Work out the finished part from the listing and answer in its coordinate system (mm). Round coordinates to 2 decimals unless told otherwise and drop trailing zeros. Write each loop counter-clockwise with the first axis right and the second up, starting at its lowest first coordinate (ties: lowest second). Pieces come first, ordered by that corner, then holes. Notation, with made-up numbers: (36.25, -20) - (40.25, -20) arc R33 cw to (40.25, 8) - close; hole circle Ø10 at (44.5, 49). An arc over 180 degrees is marked (long way). Write item = value, one per line. Start each with the question number.
from build123d import *

# Parameters (mm, degrees)
SKETCH1_W           = 51
SKETCH1_H           = 46
BOSS_EXTRUDE1_DEPTH = 11
FILLET2_R           = 5.5
FILLET3_R           = 5.5


with BuildPart() as part:
    # Sketch1 → Boss-Extrude1 (new body)
    with BuildSketch(Plane.XY):
        Rectangle(SKETCH1_W, SKETCH1_H)
    extrude(amount=BOSS_EXTRUDE1_DEPTH)

    # Fillet2
    fillet2_edges = [part.edges().sort_by_distance(p)[0] for p in [
        (25.5, 0, 11),
    ]]
    fillet(fillet2_edges, radius=FILLET2_R)

    # Fillet3
    fillet3_edges = [part.edges().sort_by_distance(p)[0] for p in [
        (-25.5, 0, 11),
        (-25.5, 0, 0),
        (25.5, 0, 0),
    ]]
    fillet(fillet3_edges, radius=FILLET3_R - 0.0001)  # a hair under: the kernel refuses the full size


solid = part.part
1. Find section C-C on z = 8.75. Give the vertices of the cut face in (x, y).
2. Find section B-B on x = -21.5. Give the vertices of the cut face in (y, z), plus the area to 3 significant figures.
3. Consider line 1 (X direction, y = 8, z = 5.25); line 2 (X direction, y = -4, z = 4.25); line 3 (Z direction, x = 21, y = -4). Determine where each line is inside the solid, lowest interval first.
4. Each of these flat-tipped pins is pushed along its axis until it touches: pin 1 (4 mm diameter, centred on y = 3.5, z = 1.5, fed in from +X); pin 2 (3 mm diameter, centred on y = -16.5, z = 6.5, fed in from -X). Where does it stop, or does it pass through?
Answer key:
q1.outline = (-24.44, -23) - (24.44, -23) - (24.44, 23) - (-24.44, 23) - close
q2.outline = (-23, 0.21) - (23, 0.21) - (23, 10.79) - (-23, 10.79) - close
q2.area = 487 mm²
q3.line_1 = -25.49 to 25.49
q3.line_2 = -25.36 to 25.36
q3.line_3 = 0.09 to 10.91
q4.pin_1 = 25.12
q4.pin_2 = -25.5
